Part print with two shaded views. Sizes in mm from the minimum x, y, z corner. A direction names the side the tool comes from. Round coordinates to 2 decimals unless told otherwise and drop trailing zeros. Put each result on its own line as item: value.
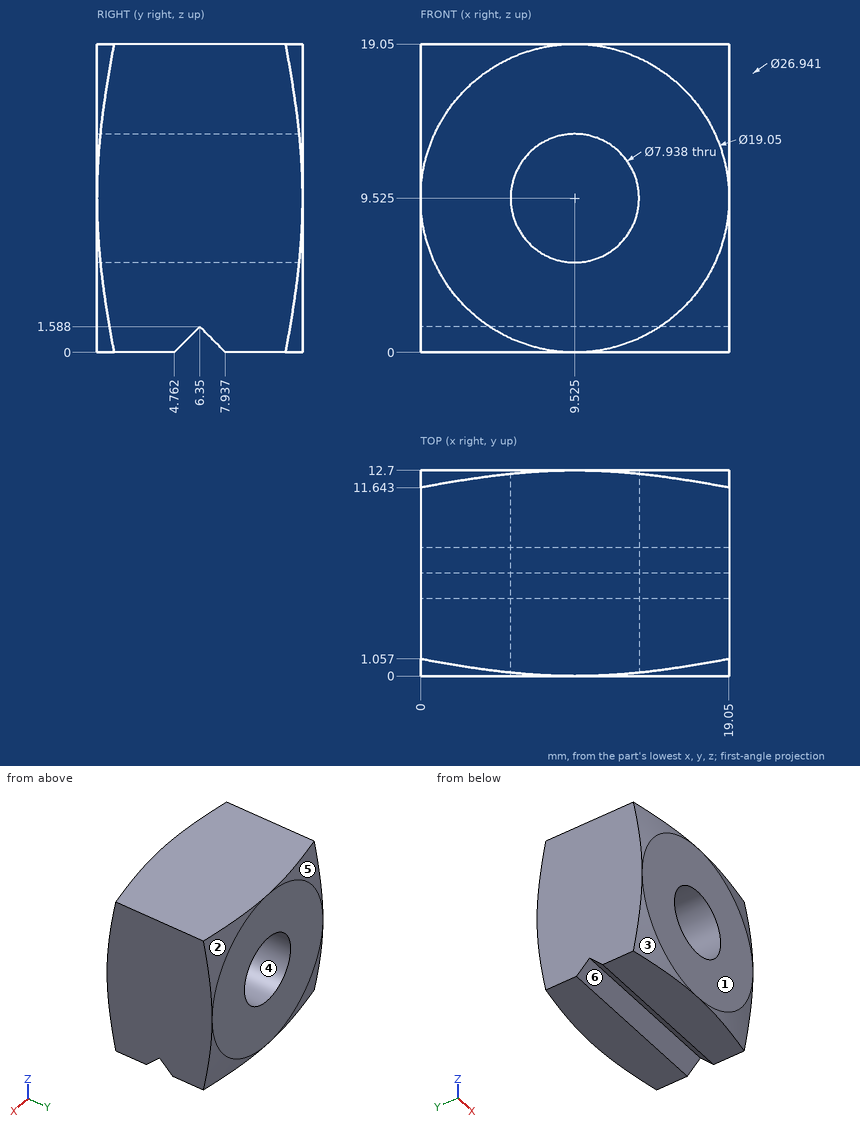
Item 1: Pin check, flat tips, straight feed: P1, Ø3, axis at x = 3.5, z = 14, coming from the -Y side; P2, Ø7, axis at x = 9.525, z = 9.525, coming from the +Y side. Stop position of each tip, or through.
Answers below:
P1: y = 0
P2: through
Item 2: Probe line 1 along Z through (x, y) = (11.25, 11.75); line 2 along X through (y, z) = (7.75, 10.75); line 3 along Z through (x, y) = (10.5, 10.5). List the from-to ranges inside material, lowest first. Write a range as [from, to].
Answers below:
line 1: [0, 5.95], [13.1, 19.05]
line 2: [0, 5.75], [13.3, 19.05]
line 3: [0, 5.68], [13.37, 19.05]
Item 3: Mould opens along Z. For the marked faces 1, 2, 3 and 4 say: pulls with the +Z half, pulls with the -Z half, needs draft (parallel to the pull), parting line crosses it, or undercut.
Answers below:
face 1: needs draft
face 2: pulls with the +Z half
face 3: pulls with the -Z half
face 4: undercut
Item 4: Tool access for the marked faces 5 and 6: list every direction of +Z, -Z, +X, -X, +Y, -Y with a clear straight run to the whole face (end or side of a thin tool).
Answers below:
face 5: +Z, -X, +Y
face 6: -Z, +X, -X
